```python
from build123d import *

# Parameters (mm, degrees)
SKETCH1_R           = 40
BOSS_EXTRUDE1_DEPTH = 10
FILLET2_R           = 2
FILLET3_R           = 4


with BuildPart() as part:
    # Sketch1 → Boss-Extrude1 (new body)
    with BuildSketch(Plane.XY):
        Circle(SKETCH1_R)
        with BuildLine():
            Line((-2.4931518, -4.318265588), (-2.4931518, -35.9135656))
            ThreePointArc((-2.4931518, -35.9135656), (-18, -31.176914536), (-29.85548425, -20.115915594))
            Line((-29.85548425, -20.115915594), (-2.4931518, -4.318265588))
        make_face(mode=Mode.SUBTRACT)
        with BuildLine():
            Line((-4.9863036, 0), (-32.34863605, -15.797650006))
            ThreePointArc((-32.34863605, -15.797650006), (-36, 0), (-32.34863605, 15.797650006))
            Line((-32.34863605, 15.797650006), (-4.9863036, 0))
        make_face(mode=Mode.SUBTRACT)
        with BuildLine():
            Line((-2.4931518, 4.318265588), (-29.85548425, 20.115915594))
            ThreePointArc((-29.85548425, 20.115915594), (-18, 31.176914536), (-2.4931518, 35.9135656))
            Line((-2.4931518, 35.9135656), (-2.4931518, 4.318265588))
        make_face(mode=Mode.SUBTRACT)
        with BuildLine():
            Line((2.4931518, 4.318265588), (2.4931518, 35.9135656))
            ThreePointArc((2.4931518, 35.9135656), (18, 31.176914536), (29.85548425, 20.115915594))
            Line((29.85548425, 20.115915594), (2.4931518, 4.318265588))
        make_face(mode=Mode.SUBTRACT)
        with BuildLine():
            Line((4.9863036, 0), (32.34863605, 15.797650006))
            ThreePointArc((32.34863605, 15.797650006), (36, 0), (32.34863605, -15.797650006))
            Line((32.34863605, -15.797650006), (4.9863036, 0))
        make_face(mode=Mode.SUBTRACT)
        with BuildLine():
            Line((2.4931518, -4.318265588), (29.85548425, -20.115915594))
            ThreePointArc((29.85548425, -20.115915594), (18, -31.176914536), (2.4931518, -35.9135656))
            Line((2.4931518, -35.9135656), (2.4931518, -4.318265588))
        make_face(mode=Mode.SUBTRACT)
        with BuildLine():
            ThreePointArc((1.539480432, 2.12), (0, -2.62), (-1.539480432, 2.12))
            Line((-1.539480432, 2.12), (1.539480432, 2.12))
        make_face(mode=Mode.SUBTRACT)
    extrude(amount=BOSS_EXTRUDE1_DEPTH)

    # Fillet2
    fillet2_edges = [part.edges().sort_by_distance(p)[0] for p in [
        (4.9863036, 0, 5),
        (2.4931518, -4.318265588, 5),
        (-2.4931518, -4.318265588, 5),
        (-4.9863036, 0, 5),
        (-2.4931518, 4.318265588, 5),
        (2.4931518, 4.318265588, 5),
    ]]
    fillet(fillet2_edges, radius=FILLET2_R)

    # Fillet3
    fillet3_edges = [part.edges().sort_by_distance(p)[0] for p in [
        (32.34863605, 15.797650006, 5),
        (32.34863605, -15.797650006, 5),
        (29.85548425, -20.115915594, 5),
        (2.4931518, -35.9135656, 5),
        (-2.4931518, -35.9135656, 5),
        (-29.85548425, -20.115915594, 5),
        (-32.34863605, -15.797650006, 5),
        (-32.34863605, 15.797650006, 5),
        (-29.85548425, 20.115915594, 5),
        (-2.4931518, 35.9135656, 5),
        (2.4931518, 35.9135656, 5),
        (29.85548425, 20.115915594, 5),
    ]]
    fillet(fillet3_edges, radius=FILLET3_R)


solid = part.part
```
Source: CAD feature listing. Evaluate the final solid. Frame: model axes, mm. Give positions to 0.01 mm unless a question says otherwise; leave off trailing zeros. Write each loop counter-clockwise with the first axis right and the second up, starting at its lowest first coordinate (ties: lowest second). Pieces come first, ordered by that corner, then holes.
1. Material intervals for line 1 along Y through (x, z) = (0, 5.5); line 2 along Y through (x, z) = (-22.5, 9); line 3 along Y through (x, z) = (-20, 7.25), sorted ascending.
2. Pull-direction query (Y, two-part tool) for faces 1 (the face through (-2.493, 20, 5)), 2 (the face through (-6.987, 0.029, 5.07)); classes: +Y half, -Y half, draft (parallel to the pull), parting line (faces both ways), or undercut.
3. Section query B-B (x = 0). Return the cut outline in (y, z).
4. First-contact query: pin 1 (3 mm diameter, centred on x = 29.5, z = 8, fed in from +Y); pin 2 (1 mm diameter, centred on y = -4.5, z = 6.5, fed in from -X); pin 3 (1 mm diameter, centred on y = 23.5, z = 8, fed in from -X); pin 4 (3 mm diameter, centred on x = 0, y = 0, fed in from +Z). Flat tips, straight axial feed; report the tip coordinate or a pass-through.
5. Section query C-C (y = -34). Return the cut outline in (x, z).
6. Section query D-D (x = 18). Return the cut outline in (y, z), then the cut area to 3 significant figures.
7. Section query A-A (y = 0). Return the cut outline in (x, z).
Output values:
1. line 1: y = -40 to -2.62, 2.12 to 40
1. line 2: y = -33.07 to -28.1, -15.87 to -10.11, 10.11 to 15.87, 28.1 to 33.07
1. line 3: y = -34.64 to -29.93, -14.43 to -8.67, 8.67 to 14.43, 29.93 to 34.64
2. face 1: undercut
2. face 2: undercut
3. outline: (-40, 0) - (-2.62, 0) - (-2.62, 10) - (-40, 10) - close; (2.12, 0) - (40, 0) - (40, 10) - (2.12, 10) - close
4. pin 1: stops at y = 28.57
4. pin 2: stops at x = -39.8
4. pin 3: stops at x = -32.73
4. pin 4: passes through
5. outline: (-21.07, 0) - (-11.83, 0) - (-11.83, 10) - (-21.07, 10) - close; (-3.51, 0) - (3.51, 0) - (3.51, 10) - (-3.51, 10) - close; (11.83, 0) - (21.07, 0) - (21.07, 10) - (11.83, 10) - close
6. outline: (-35.72, 0) - (-31.18, 0) - (-31.18, 10) - (-35.72, 10) - close; (-13.27, 0) - (-7.51, 0) - (-7.51, 10) - (-13.27, 10) - close; (7.51, 0) - (13.27, 0) - (13.27, 10) - (7.51, 10) - close; (31.18, 0) - (35.72, 0) - (35.72, 10) - (31.18, 10) - close
6. area: 206 mm2
7. outline: (-40, 0) - (-36, 0) - (-36, 10) - (-40, 10) - close; (-6.99, 0) - (-2.62, 0) - (-2.62, 10) - (-6.99, 10) - close; (2.62, 0) - (6.99, 0) - (6.99, 10) - (2.62, 10) - close; (36, 0) - (40, 0) - (40, 10) - (36, 10) - close
